Build history of the part. All positions in model axes, mm. A direction names the side the tool comes from. Give positions to 0.01 mm unless a question says otherwise; leave off trailing zeros. Loops run counter-clockwise (first coordinate to the right, second up) from the corner with the lowest first, then second, coordinate; pieces in that order, holes last. Notation, with made-up numbers: (-9, 59) -> (5, 59) arc R27 cw to (5, 84) -> close; hole circle Ø10 at (50, 44.25). An arc over 180 degrees is marked (long way). Answer as a JSON object with one key per item and string values. Group by question number.
Q1. Band-saw the part on B-B, the plane z = 14. Write the cut outline in (x, y), plus the area to 3 significant figures.
Q2. Wall check: probe 1 along Y at (x, z) = (0, 47); probe 2 along X at (y, z) = (38, -17); probe 3 along Y at (x, z) = (-12.5, 1). Give the ranges that are in metal, low to high. Write a range as from..to.
Q3. Tool access for faces 1 (the flat face through (-11, 9, 49.7)), 2 (the flat face through (20, -62, -34.683)): list every direction of +Z, -Z, +X, -X, +Y, -Y with a clear straight run to the whole face (end or side of a thin tool).
Q4. Band-saw the part on A-A, the plane z = -2. Write the cut outline in (x, y), plus the area to 3 significant figures.
Q5. Drop flat-ended pins along their axis: pin 1 (3 mm diameter, centred on x = 16.52, y = 0, fed in from -Z); pin 2 (1.2 mm diameter, centred on x = -16.52, y = 0, fed in from -Z); pin 3 (1.6 mm diameter, centred on x = 0, y = 16, fed in from +Z); pin 4 (8 mm diameter, centred on x = 35, y = 52.5, fed in from +Z). Give the stop position or say it passes through.
Solid Edge part; units mm, degrees
sketch "Sketch1" plane through (0, 0, 0) normal (0, -1, 0) x (1, 0, 0)
  line L0 (19, 44.7003) -> (32.3609, 21.5585)
  line L1 (32.3609, 21.5585) -> (41.921, 5)
  line L2 (41.921, 5) -> (64.832, -34.6831)
  line L3 (64.832, -34.6831) -> (69.832, -34.6831)
  line L4 (69.832, -34.6831) -> (70, -39.6803)
  line L5 (60.7889, -39.6803) -> (70, -39.6803)
  line L6 (57.8795, -34.641) -> (60.7889, -39.6803)
  line L7 (37.8795, 0) -> (57.8795, -34.641)
  line L8 (14, 41.3605) -> (37.8795, 0)
  line L9 (14, 49.7003) -> (14, 41.3605)
  line L10 (14, 49.7003) -> (19, 49.7003)
  line L11 (19, 49.7003) -> (19, 44.7003)
revolve "RevolvedProtrusion1" add sketch "Sketch1" angle 360 about axis through (0, 0, 0) along (0, 0, 1)
hole "Agujero_1" at (-16.5237, 0, 49.7003) direction (0, 0, -1) diameter 2 depth 3 thread major 2 thread length 2
pattern_circular "Pattern1" count 4 over 360 about axis through (0, 0, 49.7003) along (0, 0, -1) of "Agujero_1"
Worked answers:
{
 "1": {"outline": "circle Ø73.45 at (0, 0); hole circle Ø59.59 at (0, 0)", "area": "1,450 mm2"},
 "2": {"probe 1": "-19..-17.52, -15.52..-14, 14..15.52, 17.52..19", "probe 2": "-39.24..-28.82, 28.82..39.24", "probe 3": "-42.43..-35.15, 35.15..42.43"},
 "3": {"face 1": "+Z, +X, -X, +Y, -Y", "face 2": "+Z"},
 "4": {"outline": "circle Ø91.92 at (0, 0); hole circle Ø78.07 at (0, 0)", "area": "1,850 mm2"},
 "5": {"pin 1": "z = 34.4", "pin 2": "z = 35.96", "pin 3": "z = 49.7", "pin 4": "z = -24.75"}
}
